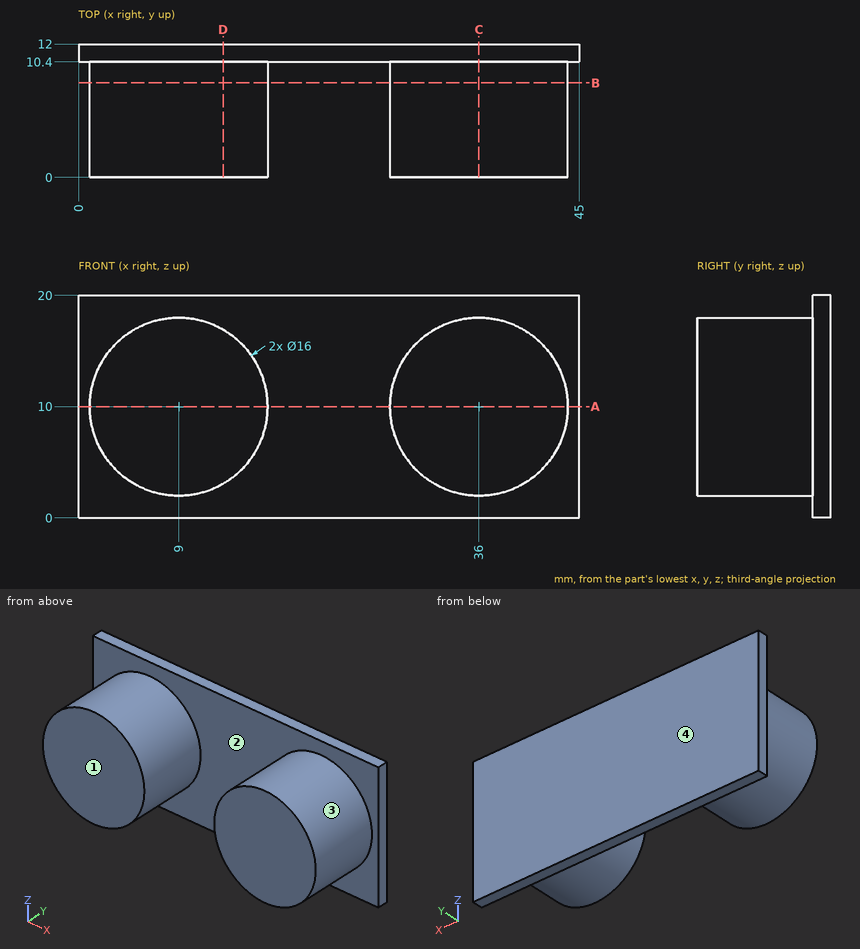
Part print with two shaded views. Sizes in mm from the minimum x, y, z corner. A direction names the side the tool comes from. Coordinates: 2 decimals unless noted, no trailing zeros. Order: outer loops, then holes, each group sorted by start corner. A loop starts at its lowest first (then second) coordinate and runs counter-clockwise, first axis right, second up. Notation, with made-up numbers: M -17,-17 L 20,-17 A12 ccw 20,-9 Z; hole C 12,7.5 d1. An arc over 180 degrees is marked long. One line per question, with ' | ' between items. Start each with the question number.
1. Cut at C-C (x = 36). Write the cut outline in (y, z), plus the area to 3 significant figures.
2. Flat gauge pins, fed straight in: P1, Ø1, axis at x = 14, y = 6, coming from the +Z side; P2, Ø1.5, axis at x = 13.5, y = 3, coming from the +Z side; P3, Ø1, axis at y = 2.5, z = 13, coming from the +X side. Where does each tip first touch, or does it go through?
3. Wall check: line 1 along X through (y, z) = (1, 10); line 2 along Y through (x, z) = (26, 11); line 3 along X through (y, z) = (2.75, 14.25). Give the ranges that are in metal, low to high. Write a range as [from, to].
4. Tool access for the marked faces 1 and 2: list every direction of +Z, -Z, +X, -X, +Y, -Y with a clear straight run to the whole face (end or side of a thin tool).
5. Cut at B-B (y = 8.5). Write the cut outline in (x, z), plus the area to 3 significant figures.
6. Cut at D-D (x = 13). Write the cut outline in (y, z).
7. Cut at A-A (z = 10). Write the cut outline in (x, y).
8. Mould opens along X. For the marked faces 3 and 4 say: +X half, -X half, draft (parallel to the pull), parting line (faces both ways), or undercut.
The answers:
1) outline: M 0,2 L 10.4,2 L 10.4,0 L 12,0 L 12,20 L 10.4,20 L 10.4,18 L 0,18 Z | area: 198 mm2
2) P1: stops at z = 16.61 | P2: stops at z = 17.07 | P3: stops at x = 43.6
3) line 1: x = [1, 17], [28, 44] | line 2: y = [10.4, 12] | line 3: x = [2.22, 15.78], [29.22, 42.78]
4) face 1: +Z, -Z, +X, -X, -Y | face 2: -Y
5) outline: C 9,10 d16; C 36,10 d16 | area: 402 mm2
6) outline: M 0,3.07 L 10.4,3.07 L 10.4,0 L 12,0 L 12,20 L 10.4,20 L 10.4,16.93 L 0,16.93 Z
7) outline: M 0,10.4 L 1,10.4 L 1,0 L 17,0 L 17,10.4 L 28,10.4 L 28,0 L 44,0 L 44,10.4 L 45,10.4 L 45,12 L 0,12 Z
8) face 3: undercut | face 4: draft
